from build123d import *

# Parameters (mm, degrees)
F2_R    = 0.5
F3_SIZE = 0.5


with BuildPart() as f1:
    # F0 (on Front) → F1 (revolve)
    with BuildSketch(Plane.XZ):
        Polygon((-4.7, 0), (-3.5, 0), (0, 22), (0, 25.771429), (-0.6, 25.771429), align=None)
    revolve(axis=Axis((0, 0, 14.771429), (0, 0, 1)))

    # F2
    f2_edges = [f1.edges().sort_by_distance(p)[0] for p in [
        (0.6, 0, 25.771429),
    ]]
    fillet(f2_edges, radius=F2_R)

    # F3
    f3_edges = [f1.edges().sort_by_distance(p)[0] for p in [
        (3.5, 0, 0),
    ]]
    chamfer(f3_edges, length=F3_SIZE)


solid = f1.part
Read the model definition and answer for the solid it produces. Units are mm, in the model's axes. Round coordinates to 2 decimals unless told otherwise and drop trailing zeros. Order: outer loops, then holes, each group sorted by start corner. A loop starts at its lowest first (then second) coordinate and runs counter-clockwise, first axis right, second up.
1) The part is cut by section A-A on z = 7.25. Write down the section's boundary in (x, y).
2) Straight lines are drawn through the part: L1, parallel to Y at x = -0.25, z = 13.5; L2, parallel to Y at x = 0, z = 12.75; L3, parallel to X at y = -0.25, z = 9.75. For each, find the intervals that lie inside material, in ascending order.
3) The part is cut by section B-B on z = 23.5. Write down the section's boundary in (x, y).
4) The mould has two halves that part along Y. Classify faces 1 (the face through (0.588, 2.647, 12.498)), 2 (the face through (-2, -4, 0)), 3 (the face through (1.24, -1.14, 11.4)): released by +Y, released by -Y, zero draft, split by the parting line, or undercut.
5) The part is cut by section C-C on z = 19. Write down the section's boundary in (x, y).
6) Flat-ended cylindrical pins translate along their axes: pin 1 (1.5 mm diameter, centred on y = -1.5, z = 9.5, fed in from -X); pin 2 (2 mm diameter, centred on y = 2, z = 21.5, fed in from +X); pin 3 (1 mm diameter, centred on y = 0.5, z = 17, fed in from +X); pin 4 (1 mm diameter, centred on x = 3.5, z = 16.5, fed in from -Y). Find the tip coordinate at first contact, or state that the pin passes through.
Resolved:
1. outline: circle Ø7.09 at (0, 0); hole circle Ø4.69 at (0, 0)
2. L1: y = -2.54 to -1.33, 1.33 to 2.54
2. L2: y = -2.67 to -1.47, 1.47 to 2.67
2. L3: x = -3.14 to -1.93, 1.93 to 3.14
3. outline: circle Ø1.92 at (0, 0)
4. face 1: split by the parting line
4. face 2: zero draft
4. face 3: undercut
5. outline: circle Ø3.35 at (0, 0); hole circle Ø0.95 at (0, 0)
6. pin 1: stops at x = -3.14
6. pin 2: stops at x = 0.82
6. pin 3: stops at x = 2.05
6. pin 4: passes through
